Verification items for the finished model (mm, model axes). A direction names the side the tool comes from. Give positions to 0.01 mm unless a question says otherwise; leave off trailing zeros. Order: outer loops, then holes, each group sorted by start corner. A loop starts at its lowest first (then second) coordinate and runs counter-clockwise, first axis right, second up.
Autodesk Inventor part; units mm, degrees
ref_plane "YZ Plane" through (0, 0, 0) normal (1, 0, 0) x (0, 1, 0)
ref_plane "XZ Plane" through (0, 0, 0) normal (0, 1, 0) x (-1, 0, 0)
ref_plane "XY Plane" through (0, 0, 0) normal (0, 0, 1) x (1, 0, 0)
sketch "Sketch1" plane through (0, 0, 0) normal (0, 1, 0) x (-1, 0, 0)
  line L0 (0, 0) -> (100, 0)
  line L1 (100, 0) -> (100, -20)
  line L2 (100, -20) -> (0, -20)
  line L3 (0, -20) -> (0, 0)
  dimension "d0" = 100
  dimension "d1" = 20
extrude "Extrusion1" add sketch "Sketch1" along normal blind 25
sketch "Sketch2" plane through (-100, 0, 0) normal (0, 0, 1) x (1, 0, 0)
  point P0 (100, 0)
sketch "Sketch3" plane through (-100, 0, 0) normal (0, 0, 1) x (1, 0, 0)
  line L0 (0, 25) -> (100, 25)
  circle A0 centre (10.25, 12.5) radius 7.5
  circle A1 centre (89.75, 12.5) radius 7.5
  point P0 (100, 0)
  dimension "d7" = 15
  dimension "d8" = 15
extrude "Extrusion2" cut sketch "Sketch3" against normal blind 20
sketch "Sketch4" plane through (-100, 0, 0) normal (0, 0, 1) x (1, 0, 0)
  point P0 (100, 0)
sketch "Sketch5" plane through (-100, 0, 0) normal (0, 0, 1) x (1, 0, 0)
  line L0 (100, 25) -> (0, 25)
  line L1 (0, 25) -> (100, 25)
  line L2 (43, 8) -> (48, 8)
  line L3 (48, 8) -> (38, 8)
  line L4 (38, 8) -> (38, 10)
  line L5 (38, 10) -> (48, 10)
  line L6 (48, 10) -> (48, 8)
  point P0 (100, 0)
  dimension "d27" = 5
  dimension "d30" = 10
extrude "Extrusion3" add sketch "Sketch5" along normal blind 10
sketch "Sketch7" plane through (-62, 10, 0) normal (0, 1, 0) x (1, 0, 0)
  line L0 (0, -10) -> (10, -10)
  circle A0 centre (5, -5) radius 2
  point P0 (62, 0)
  dimension "d32" = 4
extrude "Extrusion5" cut sketch "Sketch7" against normal blind 2
sketch "Sketch8" plane through (0, 25, 0) normal (0, 1, 0) x (1, 0, 0)
  line L0 (0, 0) -> (0, 20)
  circle A0 centre (-60, 10) radius 1.75
  circle A1 centre (-40, 10) radius 1.75
  dimension "d37" = 3.5
  dimension "d38" = 3.5
extrude "Extrusion6" cut sketch "Sketch8" against normal blind 25
properties part number "g_griper side"
(1) Section check A-A, the plane z = -10. Enter the section's corners in (x, y).
Solved:
outline: (-100, 0) - (-61.75, 0) - (-61.75, 25) - (-100, 25) - close; (-58.25, 0) - (-41.75, 0) - (-41.75, 25) - (-58.25, 25) - close; (-38.25, 0) - (0, 0) - (0, 25) - (-38.25, 25) - close; hole circle Ø15 at (-89.75, 12.5); hole circle Ø15 at (-10.25, 12.5)
(2) Section check D-D, the plane z = 5. Enter the section's corners in (x, y).
Solved:
outline: (-62, 8) - (-59, 8) - (-59, 10) - (-62, 10) - close; (-55, 8) - (-52, 8) - (-52, 10) - (-55, 10) - close
(3) Section check C-C, the plane y = 18.25. Enter the section's corners in (x, z), then the cut area to 3 significant figures.
Solved:
outline: (-100, -20) - (-94.57, -20) - (-94.57, 0) - (-100, 0) - close; (-84.93, -20) - (-15.07, -20) - (-15.07, 0) - (-84.93, 0) - close; (-5.43, -20) - (0, -20) - (0, 0) - (-5.43, 0) - close; hole circle Ø3.5 at (-60, -10); hole circle Ø3.5 at (-40, -10)
area: 1,600 mm2
(4) Go/stop test with flat-tipped pins: pin 1 (12.5 mm diameter, centred on x = -32, y = 12, fed in from +Z); pin 2 (2 mm diameter, centred on y = 9.5, z = 3.5, fed in from -X); pin 3 (5 mm diameter, centred on x = -53, y = 11, fed in from +Z); pin 4 (5 mm diameter, centred on x = -58.5, z = 3, fed in from +Y). Record where each tip stops, or that it passes through.
Solved:
pin 1: stops at z = 0
pin 2: stops at x = -62
pin 3: stops at z = 10
pin 4: stops at y = 10
(5) Release check for a two-part mould opening along X. For faces 1 (the cylindrical face through (-55.153, 9.014, 5.766)), 2 (the flat face through (-52, 9, 5)), 3 (the flat face through (-59.3, 10, 4.9)), 4 (the cylindrical face through (-97.243, 12.83, -9.86)) record: pulls with the +X half, pulls with the -X half, needs draft (parallel to the pull), parting line crosses it, or undercut.
Solved:
face 1: undercut
face 2: pulls with the +X half
face 3: needs draft
face 4: undercut
(6) Set-up check for faces 5 (the flat face through (-62, 9, 5)), 6 (the flat face through (-59.3, 8, 4.9)), 7 (the cylindrical face through (-58.331, 12.675, -10.526)): record each of +Z, -Z, +X, -X, +Y, -Y from which the full face is reachable in a straight line by a thin tool's end or side.
Solved:
face 5: +Z, -X, +Y, -Y
face 6: +Z, +X, -X, -Y
face 7: +Y, -Y
(7) Scan lines: line 1 (Z direction, x = -57, y = 8.95); line 2 (Z direction, x = -40, y = 17); line 3 (X direction, y = 17.25, z = -17.25). Record each from-to range of solid material in increasing order.
Solved:
line 1: z = -20 to 3, 7 to 10
line 2: z = -20 to -11.75, -8.25 to 0
line 3: x = -100 to -95.55, -83.95 to -16.05, -4.45 to 0
(8) Section check B-B, the plane x = -40. Enter the section's corners in (y, z).
Solved:
outline: (0, -20) - (25, -20) - (25, -11.75) - (0, -11.75) - close; (0, -8.25) - (25, -8.25) - (25, 0) - (0, 0) - close
